```python
from build123d import *

# Parameters (mm, degrees)
F0_W      = 210
F0_H      = 230
F0_W_2    = 50
F0_H_2    = 10
F1_DEPTH  = 80
F2_W      = 210
F2_H      = 230
F3_DEPTH  = 10
F5_W      = 20
F5_H      = 63
F6_DEPTH  = 1
F7_W      = 19.6074382961
F7_H      = 62.4177437024
F8_DEPTH  = 60
F9_W      = 25
F9_H      = 60
F10_DEPTH = 10
F11_W     = 19.6074382961
F11_H     = 52.7124775872
F12_DEPTH = 5
F13_DEPTH = 5


with BuildPart() as f1:
    # F0 (on Top) → F1 (new body)
    with BuildSketch(Plane.XY):
        with Locations((-9.5208105445, 45.2947338848)):
            Rectangle(F0_W, F0_H)
        Polygon((-104.5208105445, -59.7052661152), (-104.5208105445, 150.2947338848), (85.4791894555, 150.2947338848), (85.4791894555, -9.7052661152), (85.4791894555, -19.7052661152), (85.4791894555, -59.7052661152), (35.4791894555, -59.7052661152), align=None, mode=Mode.SUBTRACT)
        with Locations((60.4791894555, -14.7052661152)):
            Rectangle(F0_W_2, F0_H_2)
    extrude(amount=F1_DEPTH)

    # F2 (on face) → F3 (join)
    with BuildSketch(Plane(origin=(0, 0, 0), x_dir=(1, 0, 0), z_dir=(0, 0, -1))):
        with Locations((-9.5208105445, -45.2947338848)):
            Rectangle(F2_W, F2_H)
        Polygon((-104.5208105445, -150.2947338848), (-104.5208105445, 59.7052661152), (85.4791894555, 59.7052661152), (85.4791894555, 19.7052661152), (35.4791894555, 19.7052661152), (35.4791894555, 9.7052661152), (85.4791894555, 9.7052661152), (85.4791894555, -150.2947338848), align=None, mode=Mode.SUBTRACT)
        Polygon((85.4791894555, 59.7052661152), (-104.5208105445, 59.7052661152), (-104.5208105445, -150.2947338848), (85.4791894555, -150.2947338848), (85.4791894555, 9.7052661152), (35.4791894555, 9.7052661152), (35.4791894555, 19.7052661152), (85.4791894555, 19.7052661152), align=None)
    extrude(amount=F3_DEPTH)

    # F5 (on offset) → F6 (join)
    with BuildSketch(Plane.XY.offset(60)):
        Polygon((85.6644883752, 150.4975861311), (-104.3355116248, 150.4975861311), (-104.3355116248, 120.4975861311), (-74.7061234713, 120.4975861311), (55.8717511594, 120.4975861311), (85.6644883752, 120.4975861311), align=None)
        Polygon((-74.7061234713, 120.4975861311), (-104.3355116248, 120.4975861311), (-104.7061234713, 120.4975861311), (-104.7061234713, 40.4975861311), (-74.7061234713, 40.4975861311), align=None)
        Polygon((85.8717511594, 120.4975861311), (85.6644883752, 120.4975861311), (55.8717511594, 120.4975861311), (55.8717511594, 52.7124775872), (65.8717511594, 52.7124775872), (85.8717511594, 52.7124775872), align=None)
        with Locations((75.8717511594, 21.2124775872)):
            Rectangle(F5_W, F5_H)
    extrude(amount=F6_DEPTH)

    # F7 (on face) → F8 (join)
    with BuildSketch(Plane.XY.offset(61)):
        with Locations((75.6754703075, 21.503605736)):
            Rectangle(F7_W, F7_H)
    extrude(amount=-F8_DEPTH)

    # F9 (on face) → F10 (cut, through all)
    with BuildSketch(Plane.YZ.offset(95.4791894555)):
        with Locations((-42.2052661152, 30)):
            Rectangle(F9_W, F9_H)
    extrude(amount=-F10_DEPTH, mode=Mode.SUBTRACT)

    # F11 (on face) → F12 (join)
    with BuildSketch(Plane.XY.offset(61)):
        with Locations((75.6754703075, 26.3562387936)):
            Rectangle(F11_W, F11_H)
    extrude(amount=F12_DEPTH)

    # F13 (add): a face of the model
    f13_faces = [f1.faces().sort_by_distance(p)[0] for p in [
        (75.6754703075, -4.8526330576, 61),
    ]]
    extrude(f13_faces, amount=F13_DEPTH)


solid = f1.part
```
Can you work these out from the model? Positions are in its coordinate system, mm. A direction names the side the tool comes from. Round coordinates to 2 decimals unless told otherwise and drop trailing zeros. Loops run counter-clockwise (first coordinate to the right, second up) from the corner with the lowest first, then second, coordinate; pieces in that order, holes last.
Item 1: Suppose I cut it at A-A, the plane y = 0.5. Write out the boundary of the cut face in (x, z).
Item 2: Will these pins go through, and if not, where does the flat tip stop? pin 1 Ø15.5 at (x, y) = (71, 14.5) entering from +Z; pin 2 Ø4 at (x, y) = (-8.5, -13) entering from +Z; pin 3 Ø1.5 at (y, z) = (-45, 20.5) entering from +X.
Item 3: Suppose I cut it at C-C, the plane z = 45.5. Write out the boundary of the cut face in (x, y), then the cut area to 3 significant figures.
Item 4: If we mould it in two halves opening along X, with no side actions, what happens to faces 1 (the flat face through (91, -29.705, 30)), 2 (the flat face through (76, 52.712, 31)), 3 (the flat face through (95.479, 47, 36))? For each: +X half, -X half, draft (parallel to the pull), parting line (faces both ways), or undercut.
Item 5: Which directions (+Z, -Z, +X, -X, +Y, -Y) give clear straight access to the entire face, cutting with the end or side of a thin tool? Please do faces 4 (the flat face through (85.479, 89, 30)), 5 (the flat face through (-11, 44, -10)), 6 (the flat face through (91, -54.705, 30)), 7 (the flat face through (76, 22, 66)), 8 (the flat face through (-11, -69.705, 36)).
Item 6: Please list where these lines run through material, in increasing order: L1, parallel to Y at x = 78, z = 63.5; L2, parallel to Y at x = 53, z = 25; L3, parallel to Y at x = -21.5, z = 11.
Item 7: Suppose I cut it at D-D, the plane y = 44. Write out the boundary of the cut face in (x, z).
Item 8: Suppose I cut it at B-B, the plane x = -80.5. Write out the boundary of the cut face in (y, z).
Reported:
1. outline: (-114.52, -10) - (95.48, -10) - (95.48, 80) - (85.48, 80) - (85.48, 66) - (65.87, 66) - (65.87, 1) - (85.48, 1) - (85.48, 0) - (-104.52, 0) - (-104.52, 80) - (-114.52, 80) - close
2. pin 1: stops at z = 66
2. pin 2: stops at z = 0
2. pin 3: stops at x = -104.52
3. outline: (-114.52, -69.71) - (95.48, -69.71) - (95.48, -54.71) - (85.48, -54.71) - (85.48, -59.71) - (-104.52, -59.71) - (-104.52, 150.29) - (85.48, 150.29) - (85.48, 52.71) - (65.87, 52.71) - (65.87, -9.71) - (35.48, -9.71) - (35.48, -19.71) - (85.48, -19.71) - (85.48, -29.71) - (95.48, -29.71) - (95.48, 160.29) - (-114.52, 160.29) - close
3. area: 9,870 mm2
4. face 1: draft
4. face 2: undercut
4. face 3: +X half
5. face 4: none
5. face 5: -Z, +X, -X, +Y, -Y
5. face 6: +X
5. face 7: +Z
5. face 8: +Z, -Z, +X, -X, -Y
6. L1: y = -69.71 to -59.71, -19.71 to 52.71, 150.29 to 160.29
6. L2: y = -69.71 to -59.71, -19.71 to -9.71, 150.29 to 160.29
6. L3: y = -69.71 to -59.71, 150.29 to 160.29
7. outline: (-114.52, -10) - (95.48, -10) - (95.48, 80) - (85.48, 80) - (85.48, 66) - (65.87, 66) - (65.87, 1) - (85.48, 1) - (85.48, 0) - (-104.52, 0) - (-104.52, 60) - (-74.71, 60) - (-74.71, 61) - (-104.52, 61) - (-104.52, 80) - (-114.52, 80) - close
8. outline: (-69.71, -10) - (160.29, -10) - (160.29, 80) - (150.29, 80) - (150.29, 61) - (40.5, 61) - (40.5, 60) - (150.29, 60) - (150.29, 0) - (-59.71, 0) - (-59.71, 80) - (-69.71, 80) - close
